Source: three-view drawing plus pictorial views. Frame: mm from the lowest corner of the part. A direction names the side the tool comes from. Give positions to 0.01 mm unless a question says otherwise; leave off trailing zeros. Order: outer loops, then holes, each group sorted by start corner. A loop starts at its lowest first (then second) coordinate and runs counter-clockwise, first axis right, second up. Notation, with made-up numbers: (39, 54.25) - (51, 54.25) arc R25 cw to (51, 69.25) - close; hole circle Ø4 at (-11, -26.5). An arc over 180 degrees is marked (long way). Answer in a Markdown table with one row per item. Add a question column.
1. Section query D-D on y = 38.5. Return loops of the section in (x, z).
2. Access query for the marked faces 1, 2, 3, 4 and 5. Directions: +Z, -Z, +X, -X, +Y, -Y. A direction counts if a zero-diameter tool reaches every point of the face in a straight line with its end or side. Return the directions, or none.
3. Contact query for flat-ended pins moving along their axis: pin 1 (4 mm diameter, centred on x = 39.5, y = 13.5, fed in from +Z); pin 2 (1.8 mm diameter, centred on y = 9.5, z = 41.5, fed in from +X); pin 3 (17 mm diameter, centred on x = 59.5, y = 29.5, fed in from -Z). Output: stop coordinate, or through.
4. Ray query, line 1 (X direction, y = 27, z = 66.5); line 2 (Y direction, x = 52, z = 8.5). Return the intervals inside material, ascending. Write a range as [from, to].
5. Section query C-C on y = 15. Return loops of the section in (x, z), and give its area (3 significant figures).
6. Section query A-A on x = 41.5. Return loops of the section in (y, z), and give its area (3 significant figures).
7. Section query B-B on z = 41.5. Return loops of the section in (x, y).
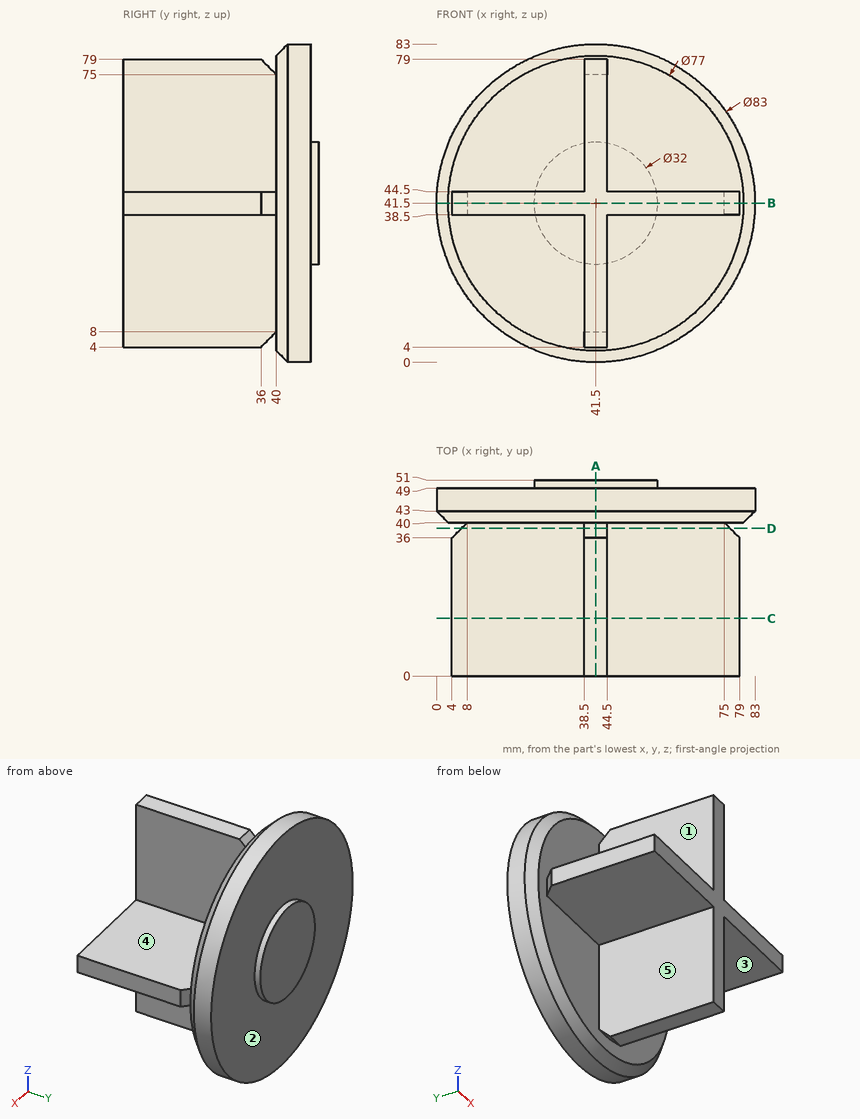
Answer:
| question | item | result |
|---|---|---|
| 1 | outline | (6.5, 38.5) - (38.5, 38.5) - (38.5, 6.5) - (44.5, 6.5) - (44.5, 38.5) - (76.5, 38.5) - (76.5, 44.5) - (44.5, 44.5) - (44.5, 76.5) - (38.5, 76.5) - (38.5, 44.5) - (6.5, 44.5) - close |
| 2 | face 1 | +Z, -X, -Y |
| 2 | face 2 | +Y |
| 2 | face 3 | -Z, +X, -Y |
| 2 | face 4 | +Z, +X, -Y |
| 2 | face 5 | -Z, -X, -Y |
| 3 | pin 1 | stops at z = 79 |
| 3 | pin 2 | stops at x = 79 |
| 3 | pin 3 | stops at z = 38.5 |
| 4 | line 1 | x = [38.5, 44.5] |
| 4 | line 2 | y = [40, 49] |
| 5 | outline | (4, 38.5) - (38.5, 38.5) - (38.5, 4) - (44.5, 4) - (44.5, 38.5) - (79, 38.5) - (79, 44.5) - (44.5, 44.5) - (44.5, 79) - (38.5, 79) - (38.5, 44.5) - (4, 44.5) - close |
| 5 | area | 864 mm² |
| 6 | outline | (0, 4) - (36, 4) - (40, 8) - (40, 3) - (43, 0) - (49, 0) - (49, 25.5) - (51, 25.5) - (51, 57.5) - (49, 57.5) - (49, 83) - (43, 83) - (40, 80) - (40, 75) - (36, 79) - (0, 79) - close |
| 6 | area | 3,790 mm² |
| 7 | outline | (0, 43) - (3, 40) - (8, 40) - (4, 36) - (4, 0) - (79, 0) - (79, 36) - (75, 40) - (80, 40) - (83, 43) - (83, 49) - (57.5, 49) - (57.5, 51) - (25.5, 51) - (25.5, 49) - (0, 49) - close |
